```python
from build123d import *

# Parameters (mm, degrees)
SKETCH1_W           = 38.1
SKETCH1_H           = 38.1
BOSS_EXTRUDE1_DEPTH = 6.35
SKETCH2_W           = 6.35
SKETCH2_H           = 38.1
BOSS_EXTRUDE2_DEPTH = 16.9418
SKETCH4_W           = 6.35
SKETCH4_H           = 38.1
BOSS_EXTRUDE3_DEPTH = 45.3898
SKETCH5_W           = 25.4
SKETCH5_H           = 38.1
BOSS_EXTRUDE4_DEPTH = 7.4549
SKETCH6_R           = 4.826
CUT_EXTRUDE1_DEPTH  = 70.299458232
SKETCH8_R           = 4.826
CUT_EXTRUDE2_DEPTH  = 69.600040729
FILLET7_R           = 2.54


with BuildPart() as part:
    # Sketch1 → Boss-Extrude1 (new body)
    with BuildSketch(Plane.XY):
        Rectangle(SKETCH1_W, SKETCH1_H)
    extrude(amount=-BOSS_EXTRUDE1_DEPTH)

    # Sketch2 → Boss-Extrude2 (add)
    with BuildSketch(Plane(origin=(0, 0, -6.35), x_dir=(-1, 0, 0), z_dir=(0, 0, -1))):
        with Locations((-15.875, 0)):
            Rectangle(SKETCH2_W, SKETCH2_H)
    extrude(amount=BOSS_EXTRUDE2_DEPTH)

    # Sketch4 → Boss-Extrude3 (add)
    with BuildSketch(Plane(origin=(19.05, 0, 0), x_dir=(0, 0, -1), z_dir=(1, 0, 0))):
        with Locations((20.1168, 0)):
            Rectangle(SKETCH4_W, SKETCH4_H)
    extrude(amount=BOSS_EXTRUDE3_DEPTH)

    # Sketch5 → Boss-Extrude4 (add)
    with BuildSketch(Plane.XY.offset(-16.9418)):
        with Locations((51.7398, 0)):
            Rectangle(SKETCH5_W, SKETCH5_H)
    extrude(amount=BOSS_EXTRUDE4_DEPTH)

    # Sketch6 → Cut-Extrude1 (cut, through all)
    with BuildSketch(Plane(origin=(0, 0, -6.35), x_dir=(-1, 0, 0), z_dir=(0, 0, -1))):
        with Locations((6.35, 9.525)):
            Circle(SKETCH6_R)
        with Locations(Location((6.35, -9.525, 0), (0, 0, 180))):
            Circle(SKETCH6_R)
    extrude(amount=-CUT_EXTRUDE1_DEPTH, mode=Mode.SUBTRACT)

    # Sketch8 → Cut-Extrude2 (cut, through all)
    with BuildSketch(Plane.XY.offset(-9.4869)):
        with Locations((51.7398, -9.525)):
            Circle(SKETCH8_R)
        with Locations(Location((51.7398, 9.525, 0), (0, 0, 180))):
            Circle(SKETCH8_R)
    extrude(amount=-CUT_EXTRUDE2_DEPTH, mode=Mode.SUBTRACT)

    # Fillet7
    fillet7_edges = [part.edges().sort_by_distance(p)[0] for p in [
        (-19.05, 0, -6.35),
        (12.7, 0, -6.35),
        (12.7, 0, -23.2918),
        (64.4398, 0, -23.2918),
    ]]
    fillet(fillet7_edges, radius=FILLET7_R)


solid = part.part
```
The listing builds one solid part. Answer for the finished solid, in the listing's coordinates (mm). A direction names the side the tool comes from. Coordinates: 2 decimals unless noted, no trailing zeros. Loops run counter-clockwise (first coordinate to the right, second up) from the corner with the lowest first, then second, coordinate; pieces in that order, holes last. Notation, with made-up numbers: (-8, 65.5) - (4, 65.5) arc R33 cw to (4, 101.5) - close; hole circle Ø8 at (29.25, 56). An arc over 180 degrees is marked (long way). Write item = value, one per line.
1) Section C-C (z = -5.5) is taken. Determine the outline of the cut face in (x, y) (3 decimals).
Responses:
outline = (-18.406, -19.05) - (19.05, -19.05) - (19.05, 19.05) - (-18.406, 19.05) - close; hole circle Ø9.652 at (-6.35, -9.525); hole circle Ø9.652 at (-6.35, 9.525)
2) Section B-B (y = -0.5) is taken. Determine the outline of the cut face in (x, z).
Responses:
outline = (-19.05, -3.81) arc R2.54 ccw to (-16.51, -6.35) - (10.16, -6.35) arc R2.54 cw to (12.7, -8.89) - (12.7, -20.75) arc R2.54 ccw to (15.24, -23.29) - (61.9, -23.29) arc R2.54 ccw to (64.44, -20.75) - (64.44, -9.49) - (39.04, -9.49) - (39.04, -16.94) - (19.05, -16.94) - (19.05, 0) - (-19.05, 0) - close
3) Which of the six approach directions +Z, -Z, +X, -X, +Y, -Y give full straight-line access (tool end or side, diameter ignored) to faces 5 (the face through (12.7, 0, -15)), 6 (the face through (38, 0, -23.292)), 7 (the face through (52, 0, -9.487)), 8 (the face through (19.05, 0, -8)), 9 (the face through (-19.05, 0, -2))?
Responses:
face_5 = -Z, -X, +Y, -Y
face_6 = -Z, +X, -X, +Y, -Y
face_7 = +Z, +X, +Y, -Y
face_8 = +Z, +Y, -Y
face_9 = +Z, -Z, -X, +Y, -Y
4) Determine the mould class of faces 1 (the face through (-1.89, -7.68, -3.22)), 2 (the face through (31, -19.05, -20)), 3 (the face through (31, 19.05, -20)), 4 (the face through (64.44, 0, -15)) for opening direction Y: pulls with the +Y half, pulls with the -Y half, needs draft (parallel to the pull), parting line crosses it, or undercut.
Responses:
face_1 = undercut
face_2 = pulls with the -Y half
face_3 = pulls with the +Y half
face_4 = needs draft
5) Find the intervals of material crossed by line 1 along X through (y, z) = (16.5, -10.75); line 2 along Y through (x, z) = (-8, -4); line 3 along X through (y, z) = (-7, -14.5), in increasing order.
Responses:
line_1 = 12.7 to 19.05, 39.04 to 64.44
line_2 = -19.05 to -14.06, -4.99 to 4.99, 14.06 to 19.05
line_3 = 12.7 to 19.05, 39.04 to 47.63, 55.85 to 64.44
6) Section D-D (y = -11.5) is taken. Determine the outline of the cut face in (x, z).
Responses:
outline = (-19.05, -3.81) arc R2.54 ccw to (-16.51, -6.35) - (-10.75, -6.35) - (-10.75, 0) - (-19.05, 0) - close; (-1.95, -6.35) - (10.16, -6.35) arc R2.54 cw to (12.7, -8.89) - (12.7, -20.75) arc R2.54 ccw to (15.24, -23.29) - (47.34, -23.29) - (47.34, -9.49) - (39.04, -9.49) - (39.04, -16.94) - (19.05, -16.94) - (19.05, 0) - (-1.95, 0) - close; (56.14, -23.29) - (61.9, -23.29) arc R2.54 ccw to (64.44, -20.75) - (64.44, -9.49) - (56.14, -9.49) - close
7) Each of these flat-tipped pins is pushed along its axis until it touches: P1, Ø12.5, axis at x = -6.35, y = 9.525, coming from the -Z side; P2, Ø2, axis at y = 2.5, z = -12, coming from the -X side; P3, Ø21.5, axis at x = 0, y = -3, coming from the -Z side. Where does it stop, or does it pass through?
Responses:
P1 = -6.35
P2 = 12.7
P3 = -6.42
8) Section A-A (x = -6.35) is taken. Determine the outline of the cut face in (y, z).
Responses:
outline = (-19.05, -6.35) - (-14.35, -6.35) - (-14.35, 0) - (-19.05, 0) - close; (-4.7, -6.35) - (4.7, -6.35) - (4.7, 0) - (-4.7, 0) - close; (14.35, -6.35) - (19.05, -6.35) - (19.05, 0) - (14.35, 0) - close
